Design review of the part built by this model. Coordinates are the model's own, in mm. A direction names the side the tool comes from. Coordinates: 2 decimals unless noted, no trailing zeros. Loops run counter-clockwise (first coordinate to the right, second up) from the corner with the lowest first, then second, coordinate; pieces in that order, holes last. Notation, with made-up numbers: M 84,16.25 L 93,16.25 A18 cw 93,23.25 Z; hole C -18.5,-39 d1. An arc over 180 degrees is marked long. Put each result on its own line as item: value. Start each with the question number.
(1) Take a section at A-A, the plane z = -15.5. Give the boundary of the cut face in (x, y), then the cut area to 4 significant figures.
(2) Take a section at D-D, the plane y = -14. Give the boundary of the cut face in (x, z), then the cut area to 3 significant figures.
(3) Take a section at C-C, the plane x = -4. Give the boundary of the cut face in (y, z).
(4) Take a section at B-B, the plane y = -10. Give the boundary of the cut face in (x, z).
(5) For probe 1 along X at (y, z) = (1.8, -31.15); probe 2 along X at (y, z) = (-13.5, 8.5); probe 3 along Y at (x, z) = (13.15, 2.5), list the stretches that pass through material, from the lowest coordinate up. Write a range as [from, to].
(6) For faces 1 (the flat face through (0, 0, 12)), 2 (the flat face through (-19.88, -10.14, 12.38)), 3 (the cylindrical face through (-13.641, 1.479, 17.527)), 4 (the flat face through (0, 0, -21)), list the 3-axis set-ups (+Z, -Z, +X, -X, +Y, -Y) from which the entire face can be reached by the end or side of a thin tool; tool diameter is ignored.
(7) Clearance check with flat-ended pins moving along their axes: pin 1 (8 mm diameter, centred on x = 13.15, y = -10, fed in from -Z); pin 2 (5 mm diameter, centred on x = -15.5, z = -15.5, fed in from -Y); pin 3 (8.5 mm diameter, centred on x = 1, z = 14, fed in from -Y); pin 4 (4.5 mm diameter, centred on x = 13.15, z = -31.15, fed in from -Y). State where each tip first meets the part, or that it passes through.
(8) The part is to be moulded in two halves that separate along Y. For faces 5 (the cylindrical face through (14.3, -7.78, 1.39)), 6 (the flat face through (-17, 3, 14)), 7 (the cylindrical face through (13.26, 2.535, -33.648)), say which applies: +Y half, -Y half, draft (parallel to the pull), parting line (faces both ways), or undercut.
```python
from build123d import *

# Parameters (mm, degrees)
SKETCH1_R           = 1.5
BOSS_EXTRUDE1_DEPTH = 5
SKETCH2_R           = 2.75
CUT_EXTRUDE1_DEPTH  = 3
SKETCH3_W           = 42.3
SKETCH3_H           = 5
BOSS_EXTRUDE2_DEPTH = 20
SKETCH7_R           = 2.5
CUT_EXTRUDE4_DEPTH  = 55.03373946
SKETCH8_R           = 2.5
CUT_EXTRUDE5_DEPTH  = 53.589400073
RIB1_REACH          = 64.311
SKETCH9_WALL_W      = 153.06531809
SKETCH9_WALL_H      = 2.5


with BuildPart() as part:
    # Sketch1 → Boss-Extrude1 (new body)
    with BuildSketch(Plane(origin=(0, 0, 0), x_dir=(1, 0, 0), z_dir=(0, 1, 0))):
        Polygon((-21.15, -21.15), (21.15, -21.15), (21.15, 21.15), (21.15, 41.15), (-21.15, 41.15), (-21.15, 21.15), align=None)
        with Locations(Location((-15.5, 15.5, 0), (0, 0, 270))):
            Circle(SKETCH1_R, mode=Mode.SUBTRACT)
        with Locations(Location((15.5, 15.5, 0), (0, 0, 270))):
            Circle(SKETCH1_R, mode=Mode.SUBTRACT)
        with Locations(Location((-15.5, -15.5, 0), (0, 0, 270))):
            Circle(SKETCH1_R, mode=Mode.SUBTRACT)
        with Locations(Location((15.5, -15.5, 0), (0, 0, 270))):
            Circle(SKETCH1_R, mode=Mode.SUBTRACT)
    extrude(amount=BOSS_EXTRUDE1_DEPTH)

    # Sketch2 → Cut-Extrude1 (cut)
    with BuildSketch(Plane.XZ):
        with Locations(Location((-15.5, 15.5, 0), (0, 0, 270))):
            Circle(SKETCH2_R)
        with Locations(Location((-15.5, -15.5, 0), (0, 0, 270))):
            Circle(SKETCH2_R)
        with Locations(Location((15.5, 15.5, 0), (0, 0, 270))):
            Circle(SKETCH2_R)
        with Locations(Location((15.5, -15.5, 0), (0, 0, 270))):
            Circle(SKETCH2_R)
    extrude(amount=-CUT_EXTRUDE1_DEPTH, mode=Mode.SUBTRACT)

    # Sketch3 → Boss-Extrude2 (add)
    with BuildSketch(Plane.XZ):
        with Locations((0, 1.35)):
            Rectangle(SKETCH3_W, SKETCH3_H)
    extrude(amount=BOSS_EXTRUDE2_DEPTH)

    # Sketch7 → Cut-Extrude4 (cut, through all)
    with BuildSketch(Plane(origin=(0, 1.15, 3.85), x_dir=(1, 0, 0), z_dir=(0, 0, -1))):
        with Locations((-13.15, 11.15)):
            Circle(SKETCH7_R)
        with Locations((13.15, 11.15)):
            Circle(SKETCH7_R)
    extrude(amount=CUT_EXTRUDE4_DEPTH, mode=Mode.SUBTRACT)

    # Sketch8 → Cut-Extrude5 (cut, through all)
    with BuildSketch(Plane(origin=(0, 5, 0), x_dir=(1, 0, 0), z_dir=(0, 1, 0))):
        with Locations(Location((-13.15, 31.15, 0), (0, 0, 270))):
            Circle(SKETCH8_R)
        with Locations(Location((13.15, 31.15, 0), (0, 0, 270))):
            Circle(SKETCH8_R)
    extrude(amount=-CUT_EXTRUDE5_DEPTH, mode=Mode.SUBTRACT)

    # Sketch9 wall → Rib1 (add, up to next)
    with BuildSketch(Plane(origin=(-21.15, -10, 12.5), x_dir=(0, 0.756312601861, 0.65421040061), z_dir=(0, 0.65421040061, -0.756312601861)), mode=Mode.PRIVATE) as rib1_sk1:
        with Locations((0, 1.25)):
            Rectangle(SKETCH9_WALL_W, SKETCH9_WALL_H)
    rib1_tool1 = extrude(rib1_sk1.sketch, amount=RIB1_REACH, mode=Mode.PRIVATE) - part.part
    rib1 = rib1_tool1.solids().sort_by_distance((-21.15, -10, 12.5))[0]
    add(rib1)

    # Mirror1: Rib1 across plane
    add(rib1.mirror(Plane.ZY))


solid = part.part
```
Computed values:
1. outline: M -21.15,0 L -18.25,0 L -18.25,3 L -17,3 L -17,5 L -21.15,5 Z; M -14,3 L -12.75,3 L -12.75,0 L 12.75,0 L 12.75,3 L 14,3 L 14,5 L -14,5 Z; M 17,3 L 18.25,3 L 18.25,0 L 21.15,0 L 21.15,5 L 17,5 Z
1. area: 166.5 mm^2
2. outline: M -21.15,-1.15 L 21.15,-1.15 L 21.15,9.04 L 18.65,9.04 L 18.65,3.85 L -18.65,3.85 L -18.65,9.04 L -21.15,9.04 Z
2. area: 237 mm^2
3. outline: M -20,-1.15 L 0,-1.15 L 0,-41.15 L 5,-41.15 L 5,21.15 L 0,21.15 L 0,3.85 L -20,3.85 Z
4. outline: M -21.15,-1.15 L -15.65,-1.15 L -15.65,3.85 L -18.65,3.85 L -18.65,12.5 L -21.15,12.5 Z; M -10.65,-1.15 L 10.65,-1.15 L 10.65,3.85 L -10.65,3.85 Z; M 15.65,-1.15 L 21.15,-1.15 L 21.15,12.5 L 18.65,12.5 L 18.65,3.85 L 15.65,3.85 Z
5. probe 1: x = [-21.15, -15.65], [-10.65, 10.65], [15.65, 21.15]
5. probe 2: x = [-21.15, -18.65], [18.65, 21.15]
5. probe 3: y = [-20, -12.5], [-7.5, 5]
6. face 1: +Z, -Y
6. face 2: +Z, +X, -X, -Y
6. face 3: -Y
6. face 4: -Z, +X, -X, -Y
7. pin 1: stops at z = -1.15
7. pin 2: stops at y = 3
7. pin 3: stops at y = 0
7. pin 4: passes through
8. face 5: undercut
8. face 6: -Y half
8. face 7: draft
